from build123d import *

# Parameters (mm, degrees)
SKETCH1_W           = 50
SKETCH1_H           = 78.3
BOSS_EXTRUDE1_DEPTH = 2.85
SKETCH2_R           = 1.7
CUT_EXTRUDE1_DEPTH  = 47.53863986
CUT_EXTRUDE2_DEPTH  = 47.53863986
SKETCH4_W           = 10
SKETCH4_H           = 2.85
BOSS_EXTRUDE2_DEPTH = 2.85


with BuildPart() as part:
    # Sketch1 → Boss-Extrude1 (new body)
    with BuildSketch(Plane(origin=(0, 0, 0), x_dir=(1, 0, 0), z_dir=(0, 1, 0))):
        Rectangle(SKETCH1_W, SKETCH1_H)
    extrude(amount=BOSS_EXTRUDE1_DEPTH)

    # Sketch2 → Cut-Extrude1 (cut, through all)
    with BuildSketch(Plane(origin=(0, 2.85, 0), x_dir=(1, 0, 0), z_dir=(0, 1, 0))):
        with Locations(Location((7, 0, 0), (0, 0, 270))):
            Circle(SKETCH2_R)
    extrude(amount=-CUT_EXTRUDE1_DEPTH, mode=Mode.SUBTRACT)

    # Sketch3 → Cut-Extrude2 (cut, through all)
    with BuildSketch(Plane(origin=(0, 2.85, 0), x_dir=(1, 0, 0), z_dir=(0, 1, 0))):
        Polygon((-4, 35.15), (-1.7, 35.15), (-1.7, 39.15), (1.7, 39.15), (1.7, 35.15), (4, 35.15), (4, 32.15), (1.7, 32.15), (1.7, 29.15), (-1.7, 29.15), (-1.7, 32.15), (-4, 32.15), align=None)
    cut_extrude2 = extrude(amount=-CUT_EXTRUDE2_DEPTH, mode=Mode.SUBTRACT)

    # Sketch4 → Boss-Extrude2 (add)
    with BuildSketch(Plane(origin=(0, 2.85, 0), x_dir=(1, 0, 0), z_dir=(0, 1, 0))):
        with Locations((-15, 40.575)):
            Rectangle(SKETCH4_W, SKETCH4_H)
        with Locations((15, 40.575)):
            Rectangle(SKETCH4_W, SKETCH4_H)
    boss_extrude2 = extrude(amount=-BOSS_EXTRUDE2_DEPTH)

    # Mirror1: Cut-Extrude2, Boss-Extrude2 across plane
    add(cut_extrude2.mirror(Plane.XY), mode=Mode.SUBTRACT)
    add(boss_extrude2.mirror(Plane.XY))


solid = part.part
Geometry: final body of the model. Coordinates: model frame, mm. A direction names the side the tool comes from. Give positions to 0.01 mm unless a question says otherwise; leave off trailing zeros. Loops run counter-clockwise (first coordinate to the right, second up) from the corner with the lowest first, then second, coordinate; pieces in that order, holes last. Notation, with made-up numbers: M 86.25,-0.75 L 133.25,-0.75 A8 ccw 133.25,10.25 Z; hole C 13.25,27 d6. An arc over 180 degrees is marked long. Put each result on its own line as item: value. Start each with the question number.
1) Access query for faces 1 (the flat face through (-25, 1, 1)), 2 (the flat face through (20, 1, 41)), 3 (the flat face through (-6, 1, -39.15)), 4 (the flat face through (3, 1, -32.15)), 5 (the flat face through (-1.7, 1, 31)). Directions: +Z, -Z, +X, -X, +Y, -Y. A direction counts if a zero-diameter tool reaches every point of the face in a straight line with its end or side. Return the directions, or none.
2) Contact query for flat-ended pins moving along their axis: pin 1 (0.9 mm diameter, centred on y = 2, z = -40, fed in from -X); pin 2 (0.9 mm diameter, centred on x = -7.5, y = 1, fed in from +Z); pin 3 (1 mm diameter, centred on x = 1.5, y = 0.5, fed in from +Z). Output: stop coordinate, or through.
3) Cut plane A-A (x = 7). Output: boundary loops of the cut face in (y, z), then the cut area to 3 significant figures.
4) Cut plane B-B (z = 0). Output: boundary loops of the cut face in (x, y), then the cut area to 3 significant figures.
5) Pull-direction query (Z, two-part tool) for faces 6 (the flat face through (6, 1, 39.15)), 7 (the flat face through (3, 1, 35.15)), 8 (the flat face through (10, 1, -41)); classes: pulls with the +Z half, pulls with the -Z half, needs draft (parallel to the pull), parting line crosses it, or undercut.
6) Cut plane C-C (x = -6). Output: boundary loops of the cut face in (y, z), then the cut area to 3 significant figures.
7) Ray query, line 1 along X through (y, z) = (1.4, 0); line 2 along Z through (x, y) = (-4.5, 1.2); line 3 along X through (y, z) = (0.85, -37.5). Return the intervals inside material, ascending.
Verdict:
1. face 1: +Z, -Z, -X, +Y, -Y
1. face 2: +Z, +X, +Y, -Y
1. face 3: -Z, +Y, -Y
1. face 4: +Y, -Y
1. face 5: +Z, +Y, -Y
2. pin 1: x = -20
2. pin 2: z = 39.15
2. pin 3: z = 39.15
3. outline: M 0,-39.15 L 2.85,-39.15 L 2.85,-1.7 L 0,-1.7 Z; M 0,1.7 L 2.85,1.7 L 2.85,39.15 L 0,39.15 Z
3. area: 213 mm2
4. outline: M -25,0 L 5.3,0 L 5.3,2.85 L -25,2.85 Z; M 8.7,0 L 25,0 L 25,2.85 L 8.7,2.85 Z
4. area: 133 mm2
5. face 6: pulls with the +Z half
5. face 7: undercut
5. face 8: needs draft
6. outline: M 0,-39.15 L 2.85,-39.15 L 2.85,39.15 L 0,39.15 Z
6. area: 223 mm2
7. line 1: -25 to 5.3, 8.7 to 25
7. line 2: -39.15 to 39.15
7. line 3: -25 to -1.7, 1.7 to 25
